Could you check a few things on this model? Use its own coordinates, in mm. A direction names the side the tool comes from. Round coordinates to 2 decimals unless told otherwise and drop trailing zeros. Write each loop counter-clockwise with the first axis right and the second up, starting at its lowest first coordinate (ties: lowest second). Pieces come first, ordered by that corner, then holes. Notation, with made-up numbers: (53.5, 43) - (110.5, 43) arc R27 ccw to (110.5, 81) - close; hole circle Ø6 at (17.25, 49). An arc over 180 degrees is marked (long way). Put each result on its own line as item: value.
from build123d import *

# Parameters (mm, degrees)
BASE_FLANGE1_DEPTH             = 1.6
EDGE_FLANGE1_STRIP_W           = 10.4
EDGE_FLANGE1_STRIP_H           = 1.6
EDGE_FLANGE1_STRIP_CUT_DEPTH   = 41
EDGE_FLANGE1_STRIP_2_W         = 10.4
EDGE_FLANGE1_STRIP_2_H         = 1.6
EDGE_FLANGE1_STRIP_CUT_2_DEPTH = 9.5
EDGE_FLANGE1_STRIP_3_W         = 10.4
EDGE_FLANGE1_STRIP_3_H         = 1.6
EDGE_FLANGE1_STRIP_CUT_3_DEPTH = 9.5
EDGE_FLANGE1_DEPTH             = 41
EDGE_FLANGE1_BEND_DEPTH        = 9.5
EDGE_FLANGE1_BEND_2_DEPTH      = 9.5
CUT_EXTRUDE1_REACH             = 46.524
SKETCH15_R                     = 1.85
SKETCH15_R_2                   = 4
CUT_EXTRUDE2_REACH             = 53.278
SKETCH16_R                     = 1.85
CUT_EXTRUDE3_REACH             = 54.158
SKETCH17_R                     = 1.55
FILLET1_R                      = 2


# Sheet-metal steps are written as plain solids
with BuildPart() as part:
    # Sketch1 → Base-Flange1 (new body)
    with BuildSketch(Plane(origin=(0, 0, 0), x_dir=(1, 0, 0), z_dir=(0, 1, 0))):
        Polygon((-20.5, 21.15), (20.5, 21.15), (20.5, 10.65), (30, 10.65), (30, -10.65), (20.5, -10.65), (20.5, -5.65), (17.5, -5.65), (17.5, -13.65), (-17.5, -13.65), (-17.5, -5.65), (-20.5, -5.65), (-20.5, -10.65), (-30, -10.65), (-30, 10.65), (-20.5, 10.65), align=None)
    extrude(amount=BASE_FLANGE1_DEPTH)

    # Edge-Flange1 strip (across the edge) → Edge-Flange1 strip cut (cut)
    with BuildSketch(Plane(origin=(20.5, 1.6, -21.15), x_dir=(0, 0, 1), z_dir=(-1, 0, 0))):
        with Locations((-1.6, -0.8)):
            Rectangle(EDGE_FLANGE1_STRIP_W, EDGE_FLANGE1_STRIP_H)
    extrude(amount=EDGE_FLANGE1_STRIP_CUT_DEPTH, mode=Mode.SUBTRACT)

    # Edge-Flange1 strip 2 (across the edge) → Edge-Flange1 strip cut 2 (cut)
    with BuildSketch(Plane(origin=(20.5, 1.6, 10.65), x_dir=(0, 0, -1), z_dir=(1, 0, 0))):
        with Locations((-1.6, -0.8)):
            Rectangle(EDGE_FLANGE1_STRIP_2_W, EDGE_FLANGE1_STRIP_2_H)
    extrude(amount=EDGE_FLANGE1_STRIP_CUT_2_DEPTH, mode=Mode.SUBTRACT)

    # Edge-Flange1 strip 3 (across the edge) → Edge-Flange1 strip cut 3 (cut)
    with BuildSketch(Plane(origin=(-30, 1.6, 10.65), x_dir=(0, 0, -1), z_dir=(1, 0, 0))):
        with Locations((-1.6, -0.8)):
            Rectangle(EDGE_FLANGE1_STRIP_3_W, EDGE_FLANGE1_STRIP_3_H)
    extrude(amount=EDGE_FLANGE1_STRIP_CUT_3_DEPTH, mode=Mode.SUBTRACT)

    # Edge-Flange1 section (across the edge) → Edge-Flange1 (add)
    with BuildSketch(Plane(origin=(20.5, 1.6, -21.15), x_dir=(0, 0, 1), z_dir=(-1, 0, 0))):
        with BuildLine():
            Line((0, 2), (0, 25.2))
            Line((0, 25.2), (1.6, 25.2))
            Line((1.6, 25.2), (1.6, 2))
            ThreePointArc((1.6, 2), (2.185786438, 0.585786438), (3.6, 0))
            Line((3.6, 0), (3.6, -1.6))
            ThreePointArc((3.6, -1.6), (1.054415588, -0.545584412), (0, 2))
        make_face()
    extrude(amount=EDGE_FLANGE1_DEPTH)

    # Edge-Flange1 section 2 (across the edge) → Edge-Flange1 bend (add)
    with BuildSketch(Plane(origin=(20.5, 1.6, 10.65), x_dir=(0, 0, -1), z_dir=(1, 0, 0))):
        with BuildLine():
            Line((0, 2), (0, 25.2))
            Line((0, 25.2), (1.6, 25.2))
            Line((1.6, 25.2), (1.6, 2))
            ThreePointArc((1.6, 2), (2.185786438, 0.585786438), (3.6, 0))
            Line((3.6, 0), (3.6, -1.6))
            ThreePointArc((3.6, -1.6), (1.054415588, -0.545584412), (0, 2))
        make_face()
    extrude(amount=EDGE_FLANGE1_BEND_DEPTH)

    # Edge-Flange1 section 3 (across the edge) → Edge-Flange1 bend 2 (add)
    with BuildSketch(Plane(origin=(-30, 1.6, 10.65), x_dir=(0, 0, -1), z_dir=(1, 0, 0))):
        with BuildLine():
            Line((0, 2), (0, 25.2))
            Line((0, 25.2), (1.6, 25.2))
            Line((1.6, 25.2), (1.6, 2))
            ThreePointArc((1.6, 2), (2.185786438, 0.585786438), (3.6, 0))
            Line((3.6, 0), (3.6, -1.6))
            ThreePointArc((3.6, -1.6), (1.054415588, -0.545584412), (0, 2))
        make_face()
    extrude(amount=EDGE_FLANGE1_BEND_2_DEPTH)

    # Sketch15 → Cut-Extrude1 (cut, up to next)
    with BuildSketch(Plane(origin=(0, 1.6, 0), x_dir=(1, 0, 0), z_dir=(0, 1, 0)), mode=Mode.PRIVATE) as cut_extrude1_sk1:
        with Locations(Location((0, 0, 0), (0, 0, 270))):
            Circle(SKETCH15_R)
    cut_extrude1_tool1 = extrude(cut_extrude1_sk1.sketch, amount=-CUT_EXTRUDE1_REACH, mode=Mode.PRIVATE) & part.part
    # Sketch15 → Cut-Extrude1 (cut, up to next)
    with BuildSketch(Plane(origin=(0, 1.6, 0), x_dir=(1, 0, 0), z_dir=(0, 1, 0)), mode=Mode.PRIVATE) as cut_extrude1_sk2:
        with Locations(Location((8, 0, 0), (0, 0, 270))):
            Circle(SKETCH15_R_2)
    cut_extrude1_tool2 = extrude(cut_extrude1_sk2.sketch, amount=-CUT_EXTRUDE1_REACH, mode=Mode.PRIVATE) & part.part
    # Sketch15 → Cut-Extrude1 (cut, up to next)
    with BuildSketch(Plane(origin=(0, 1.6, 0), x_dir=(1, 0, 0), z_dir=(0, 1, 0)), mode=Mode.PRIVATE) as cut_extrude1_sk3:
        with Locations(Location((-8, 0, 0), (0, 0, 270))):
            Circle(SKETCH15_R_2)
    cut_extrude1_tool3 = extrude(cut_extrude1_sk3.sketch, amount=-CUT_EXTRUDE1_REACH, mode=Mode.PRIVATE) & part.part
    # Sketch15 → Cut-Extrude1 (cut, up to next)
    with BuildSketch(Plane(origin=(0, 1.6, 0), x_dir=(1, 0, 0), z_dir=(0, 1, 0)), mode=Mode.PRIVATE) as cut_extrude1_sk4:
        with Locations(Location((16, 0, 0), (0, 0, 270))):
            Circle(SKETCH15_R)
    cut_extrude1_tool4 = extrude(cut_extrude1_sk4.sketch, amount=-CUT_EXTRUDE1_REACH, mode=Mode.PRIVATE) & part.part
    # Sketch15 → Cut-Extrude1 (cut, up to next)
    with BuildSketch(Plane(origin=(0, 1.6, 0), x_dir=(1, 0, 0), z_dir=(0, 1, 0)), mode=Mode.PRIVATE) as cut_extrude1_sk5:
        with Locations(Location((-16, 0, 0), (0, 0, 270))):
            Circle(SKETCH15_R)
    cut_extrude1_tool5 = extrude(cut_extrude1_sk5.sketch, amount=-CUT_EXTRUDE1_REACH, mode=Mode.PRIVATE) & part.part
    # Sketch15 → Cut-Extrude1 (cut, up to next)
    with BuildSketch(Plane(origin=(0, 1.6, 0), x_dir=(1, 0, 0), z_dir=(0, 1, 0)), mode=Mode.PRIVATE) as cut_extrude1_sk6:
        with Locations(Location((-8, 8, 0), (0, 0, 270))):
            Circle(SKETCH15_R)
    cut_extrude1_tool6 = extrude(cut_extrude1_sk6.sketch, amount=-CUT_EXTRUDE1_REACH, mode=Mode.PRIVATE) & part.part
    # Sketch15 → Cut-Extrude1 (cut, up to next)
    with BuildSketch(Plane(origin=(0, 1.6, 0), x_dir=(1, 0, 0), z_dir=(0, 1, 0)), mode=Mode.PRIVATE) as cut_extrude1_sk7:
        with Locations(Location((-8, -8, 0), (0, 0, 270))):
            Circle(SKETCH15_R)
    cut_extrude1_tool7 = extrude(cut_extrude1_sk7.sketch, amount=-CUT_EXTRUDE1_REACH, mode=Mode.PRIVATE) & part.part
    # Sketch15 → Cut-Extrude1 (cut, up to next)
    with BuildSketch(Plane(origin=(0, 1.6, 0), x_dir=(1, 0, 0), z_dir=(0, 1, 0)), mode=Mode.PRIVATE) as cut_extrude1_sk8:
        with Locations(Location((8, -8, 0), (0, 0, 270))):
            Circle(SKETCH15_R)
    cut_extrude1_tool8 = extrude(cut_extrude1_sk8.sketch, amount=-CUT_EXTRUDE1_REACH, mode=Mode.PRIVATE) & part.part
    # Sketch15 → Cut-Extrude1 (cut, up to next)
    with BuildSketch(Plane(origin=(0, 1.6, 0), x_dir=(1, 0, 0), z_dir=(0, 1, 0)), mode=Mode.PRIVATE) as cut_extrude1_sk9:
        with Locations(Location((8, 8, 0), (0, 0, 270))):
            Circle(SKETCH15_R)
    cut_extrude1_tool9 = extrude(cut_extrude1_sk9.sketch, amount=-CUT_EXTRUDE1_REACH, mode=Mode.PRIVATE) & part.part
    add(cut_extrude1_tool1.solids().sort_by_distance((0, 1.6, 0))[0], mode=Mode.SUBTRACT)
    add(cut_extrude1_tool2.solids().sort_by_distance((8, 1.6, 0))[0], mode=Mode.SUBTRACT)
    add(cut_extrude1_tool3.solids().sort_by_distance((-8, 1.6, 0))[0], mode=Mode.SUBTRACT)
    add(cut_extrude1_tool4.solids().sort_by_distance((16, 1.6, 0))[0], mode=Mode.SUBTRACT)
    add(cut_extrude1_tool5.solids().sort_by_distance((-16, 1.6, 0))[0], mode=Mode.SUBTRACT)
    add(cut_extrude1_tool6.solids().sort_by_distance((-8, 1.6, -8))[0], mode=Mode.SUBTRACT)
    add(cut_extrude1_tool7.solids().sort_by_distance((-8, 1.6, 8))[0], mode=Mode.SUBTRACT)
    add(cut_extrude1_tool8.solids().sort_by_distance((8, 1.6, 8))[0], mode=Mode.SUBTRACT)
    add(cut_extrude1_tool9.solids().sort_by_distance((8, 1.6, -8))[0], mode=Mode.SUBTRACT)

    # Sketch16 → Cut-Extrude2 (cut, up to next)
    with BuildSketch(Plane.XY.offset(10.65), mode=Mode.PRIVATE) as cut_extrude2_sk1:
        with Locations((-24, 21.75)):
            Circle(SKETCH16_R)
    cut_extrude2_tool1 = extrude(cut_extrude2_sk1.sketch, amount=-CUT_EXTRUDE2_REACH, mode=Mode.PRIVATE) & part.part
    # Sketch16 → Cut-Extrude2 (cut, up to next)
    with BuildSketch(Plane.XY.offset(10.65), mode=Mode.PRIVATE) as cut_extrude2_sk2:
        with Locations((-24, 11.75)):
            Circle(SKETCH16_R)
    cut_extrude2_tool2 = extrude(cut_extrude2_sk2.sketch, amount=-CUT_EXTRUDE2_REACH, mode=Mode.PRIVATE) & part.part
    # Sketch16 → Cut-Extrude2 (cut, up to next)
    with BuildSketch(Plane.XY.offset(10.65), mode=Mode.PRIVATE) as cut_extrude2_sk3:
        with Locations((24, 21.75)):
            Circle(SKETCH16_R)
    cut_extrude2_tool3 = extrude(cut_extrude2_sk3.sketch, amount=-CUT_EXTRUDE2_REACH, mode=Mode.PRIVATE) & part.part
    # Sketch16 → Cut-Extrude2 (cut, up to next)
    with BuildSketch(Plane.XY.offset(10.65), mode=Mode.PRIVATE) as cut_extrude2_sk4:
        with Locations((24, 11.75)):
            Circle(SKETCH16_R)
    cut_extrude2_tool4 = extrude(cut_extrude2_sk4.sketch, amount=-CUT_EXTRUDE2_REACH, mode=Mode.PRIVATE) & part.part
    add(cut_extrude2_tool1.solids().sort_by_distance((-24, 21.75, 10.65))[0], mode=Mode.SUBTRACT)
    add(cut_extrude2_tool2.solids().sort_by_distance((-24, 11.75, 10.65))[0], mode=Mode.SUBTRACT)
    add(cut_extrude2_tool3.solids().sort_by_distance((24, 21.75, 10.65))[0], mode=Mode.SUBTRACT)
    add(cut_extrude2_tool4.solids().sort_by_distance((24, 11.75, 10.65))[0], mode=Mode.SUBTRACT)

    # Sketch17 → Cut-Extrude3 (cut, up to next)
    with BuildSketch(Plane.XY.offset(-19.55), mode=Mode.PRIVATE) as cut_extrude3_sk1:
        with Locations((-10, 16.85)):
            Circle(SKETCH17_R)
    cut_extrude3_tool1 = extrude(cut_extrude3_sk1.sketch, amount=-CUT_EXTRUDE3_REACH, mode=Mode.PRIVATE) & part.part
    # Sketch17 → Cut-Extrude3 (cut, up to next)
    with BuildSketch(Plane.XY.offset(-19.55), mode=Mode.PRIVATE) as cut_extrude3_sk2:
        with Locations((10, 16.85)):
            Circle(SKETCH17_R)
    cut_extrude3_tool2 = extrude(cut_extrude3_sk2.sketch, amount=-CUT_EXTRUDE3_REACH, mode=Mode.PRIVATE) & part.part
    add(cut_extrude3_tool1.solids().sort_by_distance((-10, 16.85, -19.55))[0], mode=Mode.SUBTRACT)
    add(cut_extrude3_tool2.solids().sort_by_distance((10, 16.85, -19.55))[0], mode=Mode.SUBTRACT)

    # Fillet1
    fillet1_edges = [part.edges().sort_by_distance(p)[0] for p in [
        (20.5, 26.8, 9.85),
        (30, 26.8, 9.85),
        (-30, 26.8, 9.85),
        (-20.5, 26.8, 9.85),
        (30, 0.8, -10.65),
        (17.5, 0.8, 13.65),
        (-17.5, 0.8, 13.65),
        (-30, 0.8, -10.65),
        (20.5, 26.8, -20.35),
        (-20.5, 26.8, -20.35),
    ]]
    fillet(fillet1_edges, radius=FILLET1_R)


solid = part.part
(1) Imagine slicing it at A-A, the plane x = -24. List the corners of the cut face in (y, z) for me, then the cut area to 3 significant figures.
Values found:
outline: (0, -10.65) - (1.6, -10.65) - (1.6, 7.05) arc R2 cw to (3.6, 9.05) - (9.9, 9.05) - (9.9, 10.65) - (3.6, 10.65) arc R3.6 ccw to (0, 7.05) - close; (13.6, 9.05) - (19.9, 9.05) - (19.9, 10.65) - (13.6, 10.65) - close; (23.6, 9.05) - (26.8, 9.05) - (26.8, 10.65) - (23.6, 10.65) - close
area: 60.6 mm^2
(2) Please list where these lines run through material, in increasing order: probe 1 along X at (y, z) = (0.65, -8); probe 2 along X at (y, z) = (0.5, 0); probe 3 along X at (y, z) = (7, 10.5). Write a range as from..to.
Values found:
probe 1: x = -30..-9.85, -6.15..6.15, 9.85..30
probe 2: x = -30..-17.85, -14.15..-12, -4..-1.85, 1.85..4, 12..14.15, 17.85..30
probe 3: x = -30..-20.5, 20.5..30
(3) If we mould it in two halves opening along X, with no side actions, what happens to faces 4 (the face through (-25.364, 23, 9.861)), 5 (the face through (-29.43, 0.81, -10.05)), 6 (the face through (20.5, 10, -20)), 7 (the face through (0, 1, 13.65))? For each: pulls with the +X half, pulls with the -X half, needs draft (parallel to the pull), parting line crosses it, or undercut.
Values found:
face 4: undercut
face 5: pulls with the -X half
face 6: pulls with the +X half
face 7: needs draft
(4) For faces 1 (the face through (-19, 1, 5.65)), 2 (the face through (-14.166, 0.811, -0.241)), 3 (the face through (-20.5, 10, -20)), which set-ups out of +Z, -Z, +X, -X, +Y, -Y let a thin tool reach every point of the face, with its end or its side?
Values found:
face 1: +Z, +Y, -Y
face 2: +Y, -Y
face 3: -Z, -X, +Y, -Y
(5) Imagine slicing it at B-B, the plane y = 7.25. List the corners of the cut face in (x, z) for me, then the cut area to 3 significant figures.
Values found:
outline: (-30, 9.05) - (-20.5, 9.05) - (-20.5, 10.65) - (-30, 10.65) - close; (-20.5, -21.15) - (20.5, -21.15) - (20.5, -19.55) - (-20.5, -19.55) - close; (20.5, 9.05) - (30, 9.05) - (30, 10.65) - (20.5, 10.65) - close
area: 96.0 mm^2
(6) Imagine slicing it at D-D, the plane x = 0. List the corners of the cut face in (y, z) for me, then the cut area to 3 significant figures.
Values found:
outline: (0, -17.55) arc R3.6 ccw to (3.6, -21.15) - (26.8, -21.15) - (26.8, -19.55) - (3.6, -19.55) arc R2 cw to (1.6, -17.55) - (1.6, -1.85) - (0, -1.85) - close; (0, 1.85) - (1.6, 1.85) - (1.6, 13.65) - (0, 13.65) - close
area: 88.2 mm^2
(7) I'm going to push flat-ended pins straight in: pin 1 (4.5 mm diameter, centred on x = -24, y = 21.75, fed in from +Z); pin 2 (5 mm diameter, centred on x = 11.5, y = 10.5, fed in from +Z); pin 3 (9 mm diameter, centred on x = -8, z = 0, fed in from +Y). Where does each tip first touch, or does it pass through?
Values found:
pin 1: stops at z = 10.65
pin 2: stops at z = -19.55
pin 3: stops at y = 1.6
(8) Imagine slicing it at C-C, the plane z = 0. List the corners of the cut face in (x, y) for me, then the cut area to 3 significant figures.
Values found:
outline: (-30, 0) - (-17.85, 0) - (-17.85, 1.6) - (-30, 1.6) - close; (-14.15, 0) - (-12, 0) - (-12, 1.6) - (-14.15, 1.6) - close; (-4, 0) - (-1.85, 0) - (-1.85, 1.6) - (-4, 1.6) - close; (1.85, 0) - (4, 0) - (4, 1.6) - (1.85, 1.6) - close; (12, 0) - (14.15, 0) - (14.15, 1.6) - (12, 1.6) - close; (17.85, 0) - (30, 0) - (30, 1.6) - (17.85, 1.6) - close
area: 52.6 mm^2
